Verification items for this drawing (mm, ordinates from the low corner). Give positions to 0.01 mm unless a question says otherwise; leave off trailing zeros. Loops run counter-clockwise (first coordinate to the right, second up) from the corner with the lowest first, then second, coordinate; pieces in that order, holes last. Notation, with made-up numbers: (55, 12.5) -> (104, 12.5) arc R20 cw to (104, 16.5) -> close; hole circle Ø5 at (13, -37.5). An arc over 180 degrees is marked (long way). Answer in a Markdown table with one row per item. Add a question column.
Q1. Section check B-B on y = 47.69. Enter the section's corners in (x, z).
Q2. Material ranges on probe 1 along Y at (x, z) = (0.8, 6.1); probe 2 along Z at (x, y) = (1, 47.69), recorded low to high.
Q3. Section check A-A on z = 6.1. Enter the section's corners in (x, y), and give its area (3 significant figures).
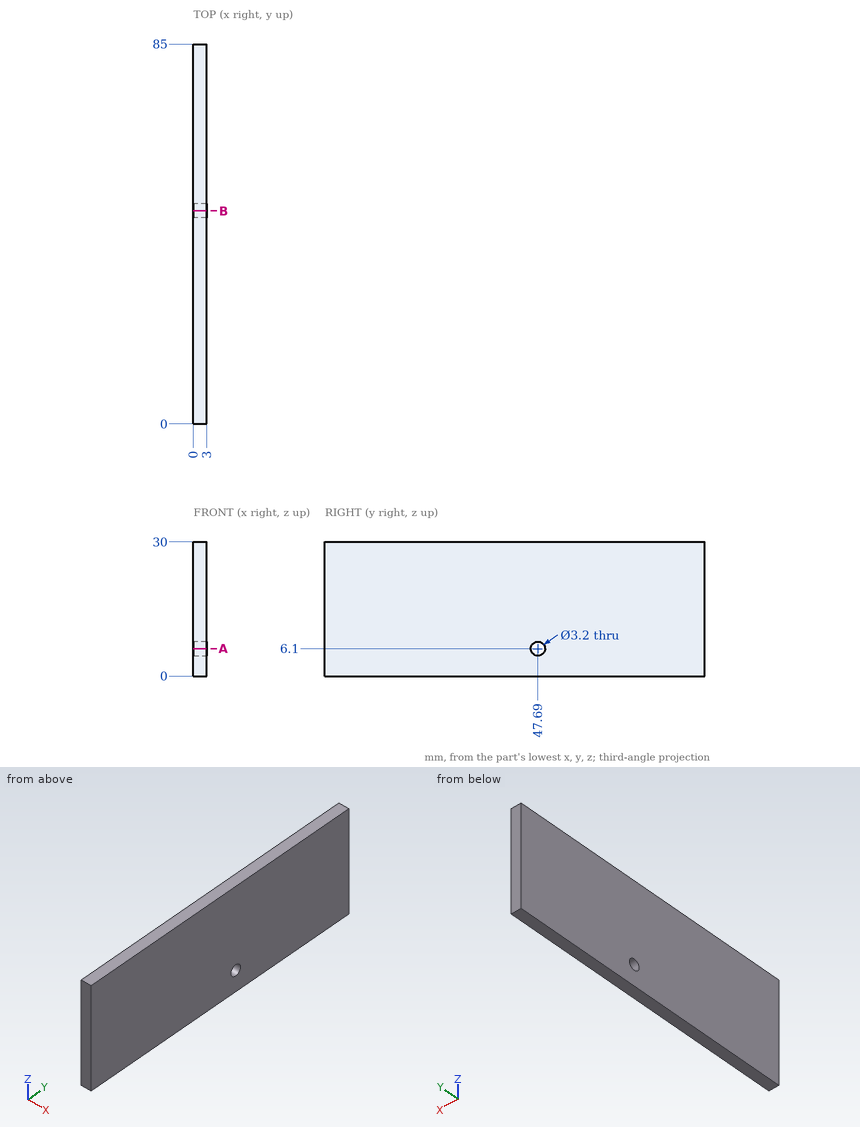
Taken from the geometry:
| question | item | result |
|---|---|---|
| 1 | outline | (0, 0) -> (3, 0) -> (3, 4.5) -> (0, 4.5) -> close; (0, 7.7) -> (3, 7.7) -> (3, 30) -> (0, 30) -> close |
| 2 | probe 1 | y = 0 to 46.09, 49.29 to 85 |
| 2 | probe 2 | z = 0 to 4.5, 7.7 to 30 |
| 3 | outline | (0, 0) -> (3, 0) -> (3, 46.09) -> (0, 46.09) -> close; (0, 49.29) -> (3, 49.29) -> (3, 85) -> (0, 85) -> close |
| 3 | area | 245 mm² |
